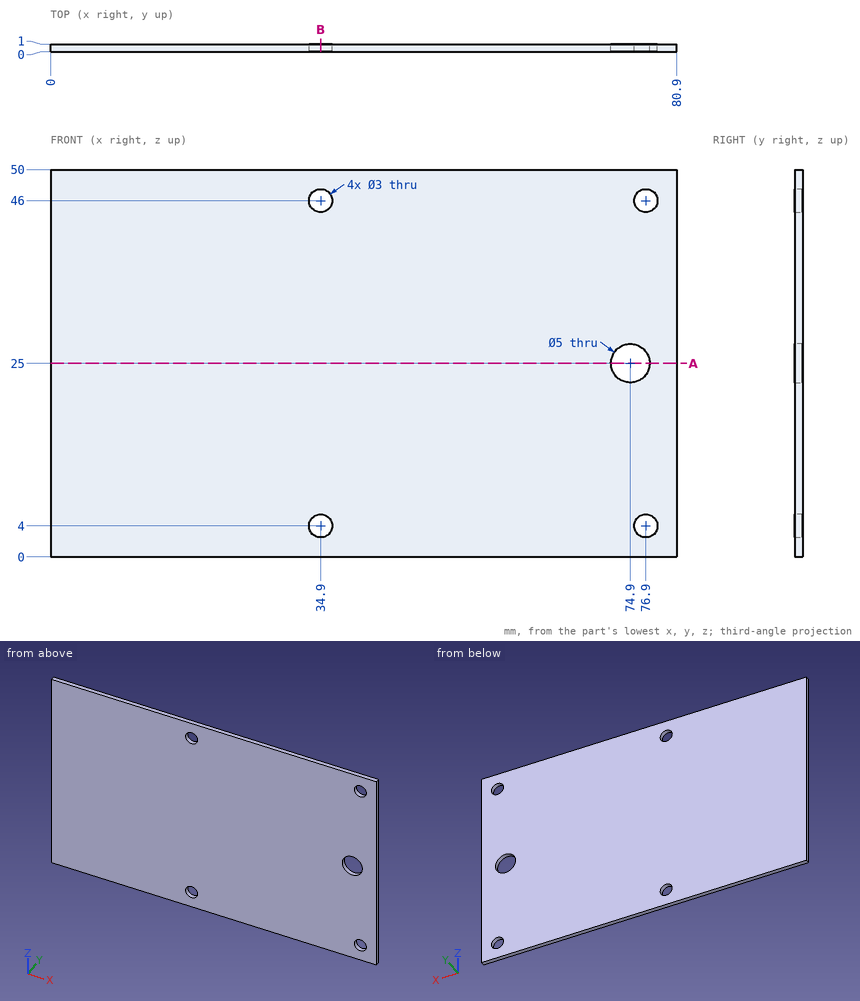
Job drawing, mm, ordinate dimensions from the low corner. One solid piece. Give positions to 0.01 mm unless a question says otherwise; leave off trailing zeros. Write each loop counter-clockwise with the first axis right and the second up, starting at its lowest first coordinate (ties: lowest second). Pieces come first, ordered by that corner, then holes. Notation, with made-up numbers: M 34.5,4 L 84.5,4 A20 cw 84.5,23 Z; hole C -28.5,52 d10. An arc over 180 degrees is marked long. One line per item, written item: value. Start each with the question number.
Q1. Drop a flat-ended pin along its axis: pin 1 Ø2.5 at (x, z) = (76.9, 46) entering from -Y. Give the stop position or say it passes through.
Q2. Saw through at B-B, the plane x = 34.9. Write the cut outline in (y, z), plus the area to 3 significant figures.
Q3. Probe probe 1 along X at (y, z) = (0.35, 46); probe 2 along X at (y, z) = (0.4, 25); probe 3 along Z at (x, y) = (76.9, 0.6). List the from-to ranges inside material, lowest first. Write a range as [from, to].
Q4. Saw through at A-A, the plane z = 25. Write the cut outline in (x, y), plus the area to 3 significant figures.
Output values:
1. pin 1: passes through
2. outline: M 0,0 L 1,0 L 1,2.5 L 0,2.5 Z; M 0,5.5 L 1,5.5 L 1,44.5 L 0,44.5 Z; M 0,47.5 L 1,47.5 L 1,50 L 0,50 Z
2. area: 44.0 mm²
3. probe 1: x = [0, 33.4], [36.4, 75.4], [78.4, 80.9]
3. probe 2: x = [0, 72.4], [77.4, 80.9]
3. probe 3: z = [0, 2.5], [5.5, 23.5], [26.5, 44.5], [47.5, 50]
4. outline: M 0,0 L 72.4,0 L 72.4,1 L 0,1 Z; M 77.4,0 L 80.9,0 L 80.9,1 L 77.4,1 Z
4. area: 75.9 mm²
